from build123d import *

# Parameters (mm, degrees)
SKETCH1_W                                           = 300
SKETCH1_H                                           = 200
BOSS_EXTRUDE1_DEPTH                                 = 10
CUT_EXTRUDE1_DEPTH                                  = 251.199920064
CUT_EXTRUDE1_DEPTH_BACK                             = 251.199920064
SKETCH2_W                                           = 33.75
SKETCH2_H                                           = 3
SKETCH3_W                                           = 200
SKETCH3_H                                           = 150
CUT_EXTRUDE2_DEPTH                                  = 4
FILLET1_R                                           = 5
CBORE_FOR_M5_HEX_SOCKET_HEAD_CAP_SCREW1_D           = 5.5
CBORE_FOR_M5_HEX_SOCKET_HEAD_CAP_SCREW1_CBORE_D     = 10
CBORE_FOR_M5_HEX_SOCKET_HEAD_CAP_SCREW1_CBORE_DEPTH = 5.4
SKETCH6_W                                           = 40
SKETCH6_H                                           = 30
CUT_EXTRUDE3_DEPTH                                  = 2
CBORE_FOR_M4_HEX_SOCKET_HEAD_CAP_SCREW1_D           = 4.5
CBORE_FOR_M4_HEX_SOCKET_HEAD_CAP_SCREW1_DEPTH       = 11.5
CBORE_FOR_M4_HEX_SOCKET_HEAD_CAP_SCREW1_CBORE_D     = 8
CBORE_FOR_M4_HEX_SOCKET_HEAD_CAP_SCREW1_CBORE_DEPTH = 4.4
CBORE_FOR_M4_HEX_SOCKET_HEAD_CAP_SCREW1_TIP         = 1.351936393


with BuildPart() as part:
    # Sketch1 → Boss-Extrude1 (new body)
    with BuildSketch(Plane(origin=(0, 0, 0), x_dir=(1, 0, 0), z_dir=(0, 1, 0))):
        Rectangle(SKETCH1_W, SKETCH1_H)
    extrude(amount=BOSS_EXTRUDE1_DEPTH)

    # Sketch2 → Cut-Extrude1 (cut, two sides: drawn at the far end of the back side and taken through both)
    with BuildSketch(Plane.XY.offset(100).offset(-CUT_EXTRUDE1_DEPTH_BACK)):
        with Locations((-133.125, 1.5)):
            Rectangle(SKETCH2_W, SKETCH2_H)
        with Locations((133.125, 1.5)):
            Rectangle(SKETCH2_W, SKETCH2_H)
    extrude(amount=CUT_EXTRUDE1_DEPTH + CUT_EXTRUDE1_DEPTH_BACK, mode=Mode.SUBTRACT)

    # Sketch3 → Cut-Extrude2 (cut)
    with BuildSketch(Plane(origin=(0, 10, 0), x_dir=(1, 0, 0), z_dir=(0, 1, 0))):
        Rectangle(SKETCH3_W, SKETCH3_H)
    extrude(amount=-CUT_EXTRUDE2_DEPTH, mode=Mode.SUBTRACT)

    # Fillet1
    fillet1_edges = [part.edges().sort_by_distance(p)[0] for p in [
        (-100, 8, 75),
        (-100, 8, -75),
        (100, 8, -75),
        (100, 8, 75),
    ]]
    fillet(fillet1_edges, radius=FILLET1_R)

    # CBORE for M5 Hex Socket Head Cap Screw1 (through all)
    with Locations(Plane(origin=(0, 10, 0), x_dir=(1, 0, 0), z_dir=(0, 1, 0))):
        with Locations((146.25, 13), (120.25, 13), (120.25, -13), (146.25, -13), (-146.25, 13), (-120.25, 13), (-146.25, -13), (-120.25, -13)):
            CounterBoreHole(CBORE_FOR_M5_HEX_SOCKET_HEAD_CAP_SCREW1_D / 2, CBORE_FOR_M5_HEX_SOCKET_HEAD_CAP_SCREW1_CBORE_D / 2, CBORE_FOR_M5_HEX_SOCKET_HEAD_CAP_SCREW1_CBORE_DEPTH)

    # Sketch6 → Cut-Extrude3 (cut)
    with BuildSketch(Plane.XZ):
        with Locations((-1.749998631, 0)):
            Rectangle(SKETCH6_W, SKETCH6_H)
    extrude(amount=-CUT_EXTRUDE3_DEPTH, mode=Mode.SUBTRACT)

    # CBORE for M4 Hex Socket Head Cap Screw1
    with Locations(Plane(origin=(0, 6, 0), x_dir=(1, 0, 0), z_dir=(0, 1, 0))):
        with Locations((13.249979912, 7.5), (13.249979912, -7.5), (-16.750020088, 7.5), (-16.750020088, -7.5)):
            CounterBoreHole(CBORE_FOR_M4_HEX_SOCKET_HEAD_CAP_SCREW1_D / 2, CBORE_FOR_M4_HEX_SOCKET_HEAD_CAP_SCREW1_CBORE_D / 2, CBORE_FOR_M4_HEX_SOCKET_HEAD_CAP_SCREW1_CBORE_DEPTH, depth=CBORE_FOR_M4_HEX_SOCKET_HEAD_CAP_SCREW1_DEPTH)
            with Locations((0, 0, -(CBORE_FOR_M4_HEX_SOCKET_HEAD_CAP_SCREW1_DEPTH + CBORE_FOR_M4_HEX_SOCKET_HEAD_CAP_SCREW1_TIP / 2))):  # 118° drill point
                Cone(0, CBORE_FOR_M4_HEX_SOCKET_HEAD_CAP_SCREW1_D / 2, CBORE_FOR_M4_HEX_SOCKET_HEAD_CAP_SCREW1_TIP, mode=Mode.SUBTRACT)


solid = part.part
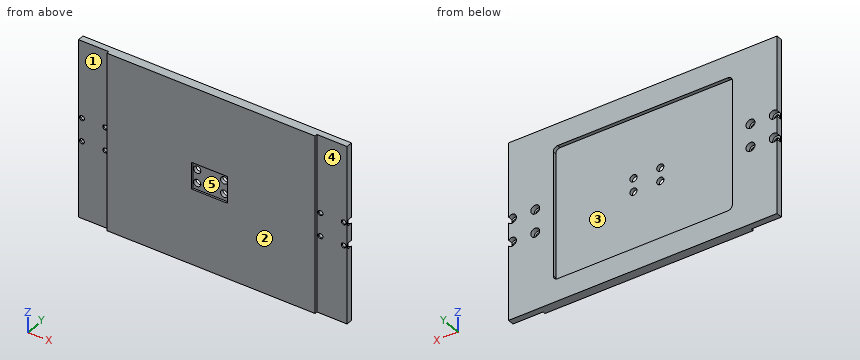
Build history of the part. All positions in model axes, mm. Face numbers are marked on the shaded views. A direction names the side the tool comes from. Give positions to 0.01 mm unless a question says otherwise; leave off trailing zeros. Order: outer loops, then holes, each group sorted by start corner. A loop starts at its lowest first (then second) coordinate and runs counter-clockwise, first axis right, second up. Notation, with made-up numbers: M 19.25,38 L 42.25,38 A17 ccw 42.25,65 Z; hole C 18,59 d6. An arc over 180 degrees is marked long. Put each result on its own line as item: value.
Item 1: Slice it at D-D, the plane z = -82.5. Write the cut outline in (x, y).
From the geometry:
outline: M -150,3 L -116.25,3 L -116.25,0 L 116.25,0 L 116.25,3 L 150,3 L 150,10 L -150,10 Z
Item 2: Two-plate mould, pull along Z, no slides. Class the marked faces 4 and 5: +Z half, -Z half, draft (parallel to the pull), parting line (faces both ways), or undercut.
From the geometry:
face 4: draft
face 5: undercut
Item 3: Probe line 1 (Z direction, x = -120.25, y = 4.05); line 2 (X direction, y = 3.85, z = -13); line 3 (Z direction, x = 2, y = 1.25). List the from-to ranges inside material, lowest first. Write a range as [from, to].
From the geometry:
line 1: z = [-100, -15.75], [-10.25, 10.25], [15.75, 100]
line 2: x = [-150, -149], [-143.5, -123], [-117.5, 117.5], [123, 143.5], [149, 150]
line 3: z = [-100, -15], [15, 100]
Item 4: Slice it at B-B, the plane x = 52.5. Write the cut outline in (y, z).
From the geometry:
outline: M 0,-100 L 10,-100 L 10,-75 L 6,-75 L 6,75 L 10,75 L 10,100 L 0,100 Z
Item 5: Slice it at C-C, the plane y = 7.5. Write the cut outline in (x, z), plus the area to 3 significant figures.
From the geometry:
outline: M -150,-100 L 150,-100 L 150,-16.31 A5 cw long 150,-9.69 L 150,9.69 A5 cw long 150,16.31 L 150,100 L -150,100 L -150,16.31 A5 cw long -150,9.69 L -150,-9.69 A5 cw long -150,-16.31 Z; hole C -120.25,-13 d10; hole C -120.25,13 d10; hole M -100,-70 A5 ccw -95,-75 L 95,-75 A5 ccw 100,-70 L 100,70 A5 ccw 95,75 L -95,75 A5 ccw -100,70 Z; hole C 120.25,-13 d10; hole C 120.25,13 d10
area: 29,400 mm2
Item 6: Slice it at A-A, the plane z = 45.5. Write the cut outline in (x, y), plus the area to 3 significant figures.
From the geometry:
outline: M -150,3 L -116.25,3 L -116.25,0 L 116.25,0 L 116.25,3 L 150,3 L 150,10 L 100,10 L 100,6 L -100,6 L -100,10 L -150,10 Z
area: 2,000 mm2
Item 7: 3-axis set-ups, long thin cutter, end or side, ignore diameter. For the marked faces 1, 2 and 3: which of +Z, -Z, +X, -X, +Y, -Y reach the whole face in a straight line?
From the geometry:
face 1: +Z, -Z, -X, -Y
face 2: +Z, -Z, +X, -X, -Y
face 3: +Y
Item 8: Flat gauge pins, fed straight in: pin 1 Ø3 at (x, z) = (-119, 15) entering from +Y; pin 2 Ø3 at (x, z) = (61, 26) entering from +Y; pin 3 Ø8 at (x, z) = (146.25, 13) entering from -Y. Where does each tip first touch, or does it go through?
From the geometry:
pin 1: stops at y = 4.6
pin 2: stops at y = 6
pin 3: stops at y = 3
